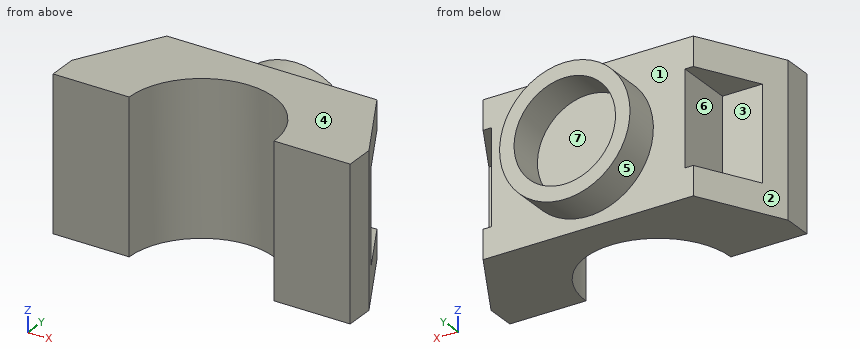
```python
from build123d import *

# Parameters (mm, degrees)
BOSS_EXTRUDE1_DEPTH = 42
SKETCH2_R           = 18
SKETCH2_R_2         = 14
BOSS_EXTRUDE2_DEPTH = 10
CUT_EXTRUDE1_DEPTH  = 26


with BuildPart() as part:
    # Sketch1 → Boss-Extrude1 (new body)
    with BuildSketch(Plane.XY):
        with BuildLine():
            Line((-30.817923278, 0), (-30.817923278, 8))
            Line((-30.817923278, 8), (-18.817923278, 30))
            Line((-18.817923278, 30), (39.182076722, 30))
            Line((39.182076722, 30), (51.182076722, 8))
            Line((51.182076722, 8), (51.182076722, 0))
            Line((51.182076722, 0), (30.182076722, 0))
            ThreePointArc((30.182076722, 0), (10.182076722, 20), (-9.817923278, 0))
            Line((-9.817923278, 0), (-30.817923278, 0))
        make_face()
    extrude(amount=-BOSS_EXTRUDE1_DEPTH)

    # Sketch2 → Boss-Extrude2 (add)
    with BuildSketch(Plane(origin=(0, 30, 0), x_dir=(1, 0, 0), z_dir=(0, 1, 0))):
        with Locations(Location((10.182076722, 21, 0), (0, 0, 270))):
            Circle(SKETCH2_R)
        with Locations(Location((10.182076722, 21, 0), (0, 0, 270))):
            Circle(SKETCH2_R_2, mode=Mode.SUBTRACT)
    extrude(amount=BOSS_EXTRUDE2_DEPTH)

    # Sketch3 → Cut-Extrude1 (cut)
    with BuildSketch(Plane.XY.offset(-8)):
        Polygon((36.909349449, 30), (36.909349449, 14), (47.909349449, 14), (39.182076722, 30), align=None)
        Polygon((-16.545196006, 30), (-16.545196006, 14), (-27.545196006, 14), (-18.817923278, 30), align=None)
    extrude(amount=-CUT_EXTRUDE1_DEPTH, mode=Mode.SUBTRACT)


solid = part.part
```
Can you work these out from the model? Positions are in its coordinate system, mm. Face numbers are marked on the shaded views. A direction names the side the tool comes from. Give positions to 0.01 mm unless a question says otherwise; leave off trailing zeros. Loops run counter-clockwise (first coordinate to the right, second up) from the corner with the lowest first, then second, coordinate; pieces in that order, holes last. Notation, with made-up numbers: M 11,65.25 L 25,65.25 A12 cw 25,73.25 Z; hole C 46.25,14.25 d11. An arc over 180 degrees is marked long. Answer in a Markdown table with one row per item.
1. Suppose I cut it at C-C on y = 18. Write out the boundary of the cut face in (x, z), plus the area to 3 significant figures.
Taken from the geometry:
| item | result |
|---|---|
| outline | M -25.36,-42 L 1.46,-42 L 1.46,0 L -25.36,0 L -25.36,-8 L -16.55,-8 L -16.55,-34 L -25.36,-34 Z; M 18.9,-42 L 45.73,-42 L 45.73,-34 L 36.91,-34 L 36.91,-8 L 45.73,-8 L 45.73,0 L 18.9,0 Z |
| area | 1,790 mm² |
2. Which directions (+Z, -Z, +X, -X, +Y, -Y) give clear straight access to the entire face, cutting with the end or side of a thin tool? Please do the marked faces 1, 2 and 3.
Taken from the geometry:
| item | result |
|---|---|
| face 1 | +Y |
| face 2 | +Z, -Z, -X, +Y |
| face 3 | -X, +Y |
3. Suppose I cut it at B-B on x = -17.5. Write out the boundary of the cut face in (y, z), plus the area to 3 significant figures.
Taken from the geometry:
| item | result |
|---|---|
| outline | M 0,-42 L 30,-42 L 30,-34 L 14,-34 L 14,-8 L 30,-8 L 30,0 L 0,0 Z |
| area | 844 mm² |
4. For pin 1 Ø5.5 at (x, z) = (-21.5, -27) entering from +Y; pin 2 Ø22.5 at (x, z) = (10.18, -21) entering from -Y; pin 3 Ø8 at (x, y) = (-6.5, 26.5) entering from +Z; pin 4 Ø2 at (x, z) = (35.5, -21) entering from +Y, each with a flat end and sliding along its axis, tell me the tip position at first contact or that it passes through.
Taken from the geometry:
| item | result |
|---|---|
| pin 1 | stops at y = 14 |
| pin 2 | stops at y = 16.53 |
| pin 3 | stops at z = 0 |
| pin 4 | stops at y = 30 |
5. Suppose I cut it at A-A on z = -21. Write out the boundary of the cut face in (x, y).
Taken from the geometry:
| item | result |
|---|---|
| outline | M -30.82,0 L -9.82,0 A20 cw 30.18,0 L 51.18,0 L 51.18,8 L 47.91,14 L 36.91,14 L 36.91,30 L 28.18,30 L 28.18,40 L 24.18,40 L 24.18,30 L -3.82,30 L -3.82,40 L -7.82,40 L -7.82,30 L -16.55,30 L -16.55,14 L -27.55,14 L -30.82,8 Z |
6. Suppose I cut it at D-D on y = 22. Write out the boundary of the cut face in (x, z), plus the area to 3 significant figures.
Taken from the geometry:
| item | result |
|---|---|
| outline | M -23.18,-42 L 43.55,-42 L 43.55,-34 L 36.91,-34 L 36.91,-8 L 43.55,-8 L 43.55,0 L -23.18,0 L -23.18,-8 L -16.55,-8 L -16.55,-34 L -23.18,-34 Z |
| area | 2,460 mm² |
7. If I drill on line 1 along X through (y, z) = (32.5, -21); line 2 along Z through (x, y) = (-24, 19); line 3 along Z through (x, y) = (2, 32), over which ranges is the centre line in solid material (lowest first)?
Taken from the geometry:
| item | result |
|---|---|
| line 1 | x = -7.82 to -3.82, 24.18 to 28.18 |
| line 2 | z = -42 to -34, -8 to 0 |
| line 3 | z = -37.03 to -32.36, -9.64 to -4.97 |
8. Thinking about a two-plate mould opening in X: for the marked faces 4, 5, 6 and 7, which applies, released by +X, released by -X, zero draft, split by the parting line, or undercut?
Taken from the geometry:
| item | result |
|---|---|
| face 4 | zero draft |
| face 5 | split by the parting line |
| face 6 | released by -X |
| face 7 | undercut |
